from build123d import *

# Parameters (mm, degrees)
EXTRUDE_DEPTH   = 4
PAD_DEPTH       = 8
POCKET_START    = 4
SKETCH001_W     = 90
SKETCH001_H     = 4
POCKET_DEPTH    = 4
POCKET001_START = -5
SKETCH002_W     = 3.5
SKETCH002_H     = 1
SKETCH002_W_2   = 2.5
SKETCH002_H_2   = 3
SKETCH002_H_3   = 1.25
POCKET001_DEPTH = 89


with BuildPart() as part:
    # Face001 → Extrude (new body)
    with BuildSketch(Plane(origin=(44.07068, 49.485801, 0), x_dir=(0, 1, 0), z_dir=(0, 0, 1))):
        with BuildLine():
            add(Edge.make_bspline(
                [(-12.189347, 20.903638), (-8.616149, 10.816398)],
                knots=[0, 0, 8.089254, 8.089254], degree=1))
            add(Edge.make_bspline(
                [(-8.616149, 10.816398), (-9.34243, 10.514773)],
                knots=[0, 0, 0.594462, 0.594462], degree=1))
            add(Edge.make_bspline(
                [(-9.34243, 10.514773), (-9.595107, 10.410263), (-9.751211, 10.165523), (-9.751211, 9.903586)],
                knots=[0, 0, 0, 0, 1, 1, 1, 1], degree=3))
            add(Edge.make_bspline(
                [(-9.751211, 9.903586), (-9.751211, 9.842732), (-9.743274, 9.781877), (-9.724753, 9.7197)],
                knots=[0, 0, 0, 0, 1, 1, 1, 1], degree=3))
            add(Edge.make_bspline(
                [(-9.724753, 9.7197), (-6.950597, 0.094159)],
                knots=[0, 0, 7.572159, 7.572159], degree=1))
            add(Edge.make_bspline(
                [(-6.950597, 0.094159), (-7.703336, -0.194237)],
                knots=[0, 0, 0.609332, 0.609332], degree=1))
            add(Edge.make_bspline(
                [(-7.703336, -0.194237), (-7.963951, -0.292133), (-8.127992, -0.542164), (-8.127992, -0.809393)],
                knots=[0, 0, 0, 0, 1, 1, 1, 1], degree=3))
            add(Edge.make_bspline(
                [(-8.127992, -0.809393), (-8.127992, -0.874216), (-8.118732, -0.939039), (-8.098888, -1.003862)],
                knots=[0, 0, 0, 0, 1, 1, 1, 1], degree=3))
            add(Edge.make_bspline(
                [(-8.098888, -1.003862), (-2.807222, -18.201779)],
                knots=[0, 0, 13.601471, 13.601471], degree=1))
            add(Edge.make_bspline(
                [(-2.807222, -18.201779), (-2.752982, -18.37905), (-2.627305, -18.524571), (-2.460617, -18.603946)],
                knots=[0, 0, 0, 0, 1, 1, 1, 1], degree=3))
            add(Edge.make_bspline(
                [(-2.460617, -18.603946), (-2.29393, -18.683321), (-2.100784, -18.689935), (-1.930128, -18.621143)],
                knots=[0, 0, 0, 0, 1, 1, 1, 1], degree=3))
            add(Edge.make_bspline(
                [(-1.930128, -18.621143), (14.607653, -12.00656)],
                knots=[0, 0, 13.46384, 13.46384], degree=1))
            add(Edge.make_bspline(
                [(14.607653, -12.00656), (14.782278, -11.936446), (14.918539, -11.796216), (14.983362, -11.620268)],
                knots=[0, 0, 0, 0, 1, 1, 1, 1], degree=3))
            add(Edge.make_bspline(
                [(14.983362, -11.620268), (15.046862, -11.444321), (15.034956, -11.248529), (14.947643, -11.083164)],
                knots=[0, 0, 0, 0, 1, 1, 1, 1], degree=3))
            add(Edge.make_bspline(
                [(14.947643, -11.083164), (6.637081, 4.667482)],
                knots=[0, 0, 13.461663, 13.461663], degree=1))
            add(Edge.make_bspline(
                [(6.637081, 4.667482), (6.480976, 4.963815), (6.127758, 5.096107), (5.815549, 4.975721)],
                knots=[0, 0, 0, 0, 1, 1, 1, 1], degree=3))
            add(Edge.make_bspline(
                [(5.815549, 4.975721), (4.96756, 4.651607)],
                knots=[0, 0, 0.686226, 0.686226], degree=1))
            add(Edge.make_bspline(
                [(4.96756, 4.651607), (-0.018513, 13.744013)],
                knots=[0, 0, 7.83859, 7.83859], degree=1))
            add(Edge.make_bspline(
                [(-0.018513, 13.744013), (-0.181232, 14.041669), (-0.541065, 14.167346), (-0.851951, 14.0377)],
                knots=[0, 0, 0, 0, 1, 1, 1, 1], degree=3))
            add(Edge.make_bspline(
                [(-0.851951, 14.0377), (-1.578232, 13.736075)],
                knots=[0, 0, 0.594462, 0.594462], degree=1))
            add(Edge.make_bspline(
                [(-1.578232, 13.736075), (-6.192565, 23.392044)],
                knots=[0, 0, 8.089595, 8.089595], degree=1))
            add(Edge.make_bspline(
                [(-6.192565, 23.392044), (-6.344701, 23.709544), (-6.717763, 23.852419), (-7.043201, 23.717482)],
                knots=[0, 0, 0, 0, 1, 1, 1, 1], degree=3))
            add(Edge.make_bspline(
                [(-7.043201, 23.717482), (-11.81893, 21.735752)],
                knots=[0, 0, 3.908466, 3.908466], degree=1))
            add(Edge.make_bspline(
                [(-11.81893, 21.735752), (-12.07293, 21.629919), (-12.227711, 21.385179), (-12.227711, 21.124565)],
                knots=[0, 0, 0, 0, 1, 1, 1, 1], degree=3))
            add(Edge.make_bspline(
                [(-12.227711, 21.124565), (-12.227711, 21.050482), (-12.215805, 20.976398), (-12.189347, 20.903638)],
                knots=[0, 0, 0, 0, 1, 1, 1, 1], degree=3))
        make_face()
        with BuildLine():
            add(Edge.make_bspline(
                [(-24.664451, 2.497898), (-24.664451, 2.132773), (-24.368117, 1.83644), (-24.002992, 1.83644)],
                knots=[0, 0, 0, 0, 1, 1, 1, 1], degree=3))
            add(Edge.make_bspline(
                [(-24.002992, 1.83644), (-15.404034, 1.83644)],
                knots=[0, 0, 6.5, 6.5], degree=1))
            add(Edge.make_bspline(
                [(-15.404034, 1.83644), (-15.404034, -1.166581)],
                knots=[0, 0, 2.27, 2.27], degree=1))
            add(Edge.make_bspline(
                [(-15.404034, -1.166581), (-24.43294, -8.905643)],
                knots=[0, 0, 8.989056, 8.989056], degree=1))
            add(Edge.make_bspline(
                [(-24.43294, -8.905643), (-24.586399, -9.036612), (-24.664451, -9.221821), (-24.664451, -9.408352)],
                knots=[0, 0, 0, 0, 1, 1, 1, 1], degree=3))
            add(Edge.make_bspline(
                [(-24.664451, -9.408352), (-24.664451, -9.560487), (-24.611534, -9.713946), (-24.504378, -9.8383)],
                knots=[0, 0, 0, 0, 1, 1, 1, 1], degree=3))
            add(Edge.make_bspline(
                [(-24.504378, -9.8383), (-24.266253, -10.116112), (-23.849534, -10.147862), (-23.571722, -9.909737)],
                knots=[0, 0, 0, 0, 1, 1, 1, 1], degree=3))
            add(Edge.make_bspline(
                [(-23.571722, -9.909737), (-14.497836, -2.13231)],
                knots=[0, 0, 9.033744, 9.033744], degree=1))
            add(Edge.make_bspline(
                [(-14.497836, -2.13231), (-12.857419, -2.13231)],
                knots=[0, 0, 1.24, 1.24], degree=1))
            add(Edge.make_bspline(
                [(-12.857419, -2.13231), (-11.318867, -2.13231), (-10.112367, -0.970789), (-10.112367, 0.513523)],
                knots=[0, 0, 0, 0, 1, 1, 1, 1], degree=3))
            add(Edge.make_bspline(
                [(-10.112367, 0.513523), (-10.112367, 4.482273)],
                knots=[0, 0, 3, 3], degree=1))
            add(Edge.make_bspline(
                [(-10.112367, 4.482273), (-10.112367, 5.990398), (-11.250076, 7.128107), (-12.758201, 7.128107)],
                knots=[0, 0, 0, 0, 1, 1, 1, 1], degree=3))
            add(Edge.make_bspline(
                [(-12.758201, 7.128107), (-14.497836, 7.128107)],
                knots=[0, 0, 1.315, 1.315], degree=1))
            add(Edge.make_bspline(
                [(-14.497836, 7.128107), (-23.571722, 14.905534)],
                knots=[0, 0, 9.033744, 9.033744], degree=1))
            add(Edge.make_bspline(
                [(-23.571722, 14.905534), (-23.848211, 15.143659), (-24.266253, 15.111909), (-24.504378, 14.834096)],
                knots=[0, 0, 0, 0, 1, 1, 1, 1], degree=3))
            add(Edge.make_bspline(
                [(-24.504378, 14.834096), (-24.611534, 14.709742), (-24.664451, 14.556284), (-24.664451, 14.404148)],
                knots=[0, 0, 0, 0, 1, 1, 1, 1], degree=3))
            add(Edge.make_bspline(
                [(-24.664451, 14.404148), (-24.664451, 14.217617), (-24.586399, 14.032409), (-24.43294, 13.902763)],
                knots=[0, 0, 0, 0, 1, 1, 1, 1], degree=3))
            add(Edge.make_bspline(
                [(-24.43294, 13.902763), (-15.404034, 6.162377)],
                knots=[0, 0, 8.989707, 8.989707], degree=1))
            add(Edge.make_bspline(
                [(-15.404034, 6.162377), (-15.404034, 3.159357)],
                knots=[0, 0, 2.27, 2.27], degree=1))
            add(Edge.make_bspline(
                [(-15.404034, 3.159357), (-24.002992, 3.159357)],
                knots=[0, 0, 6.5, 6.5], degree=1))
            add(Edge.make_bspline(
                [(-24.002992, 3.159357), (-24.368117, 3.159357), (-24.664451, 2.863023), (-24.664451, 2.497898)],
                knots=[0, 0, 0, 0, 1, 1, 1, 1], degree=3))
        make_face()
        with BuildLine():
            add(Edge.make_bspline(
                [(17.253487, -13.990935), (17.593476, -13.854675), (17.757518, -13.468383), (17.622581, -13.131039)],
                knots=[0, 0, 0, 0, 1, 1, 1, 1], degree=3))
            add(Edge.make_bspline(
                [(17.622581, -13.131039), (17.48632, -12.792373), (17.101351, -12.627008), (16.762685, -12.761946)],
                knots=[0, 0, 0, 0, 1, 1, 1, 1], degree=3))
            add(Edge.make_bspline(
                [(16.762685, -12.761946), (-3.081065, -20.699446)],
                knots=[0, 0, 16.155494, 16.155494], degree=1))
            add(Edge.make_bspline(
                [(-3.081065, -20.699446), (-3.340357, -20.803956), (-3.497784, -21.052664), (-3.497784, -21.314602)],
                knots=[0, 0, 0, 0, 1, 1, 1, 1], degree=3))
            add(Edge.make_bspline(
                [(-3.497784, -21.314602), (-3.497784, -21.396623), (-3.483232, -21.479966), (-3.450159, -21.560664)],
                knots=[0, 0, 0, 0, 1, 1, 1, 1], degree=3))
            add(Edge.make_bspline(
                [(-3.450159, -21.560664), (-3.313899, -21.899331), (-2.92893, -22.064696), (-2.590263, -21.929758)],
                knots=[0, 0, 0, 0, 1, 1, 1, 1], degree=3))
            add(Edge.make_bspline(
                [(-2.590263, -21.929758), (17.253487, -13.990935)],
                knots=[0, 0, 16.155866, 16.155866], degree=1))
        make_face()
    extrude(amount=EXTRUDE_DEPTH)


with BuildPart() as part_1:
    # Extrude placement: moved
    add(part.part.moved(Location((2.348148, 3.053205, -2))))


with BuildPart() as part_2:
    # BaseFeature placement: moved
    add(part_1.part.moved(Location((-2.348148, -3.053205, 2))))

    # Sketch → Pad (new body)
    with BuildSketch(Plane.XY):
        with BuildLine():
            Line((0, 98), (0, 5))
            ThreePointArc((0, 5), (1.464466, 1.464466), (5, 0))
            Line((5, 0), (85, 0))
            ThreePointArc((85, 0), (88.535534, 1.464466), (90, 5))
            Line((90, 5), (90, 98))
            Line((90, 98), (0, 98))
        make_face()
    extrude(amount=PAD_DEPTH)

    # Sketch001 → Pocket (cut)
    with BuildSketch(Plane.XY.offset(POCKET_START)):
        with BuildLine():
            Line((4.5, 98), (4.5, 5))
            ThreePointArc((4.5, 5), (4.792893, 4.292893), (5.5, 4))
            Line((5.5, 4), (84.5, 4))
            ThreePointArc((84.5, 4), (85.207107, 4.292893), (85.5, 5))
            Line((85.5, 5), (85.5, 98))
            Line((85.5, 98), (4.5, 98))
        make_face()
        with Locations((45, 96)):
            Rectangle(SKETCH001_W, SKETCH001_H)
    extrude(amount=POCKET_DEPTH, mode=Mode.SUBTRACT)

    # Sketch002 → Pocket001 (cut)
    with BuildSketch(Plane.XZ.offset(POCKET001_START)):
        with Locations((87.75, 4.5)):
            Rectangle(SKETCH002_W, SKETCH002_H)
        with Locations((87.75, 6.5)):
            Rectangle(SKETCH002_W_2, SKETCH002_H_2)
        with Locations((2.25, 4.375)):
            Rectangle(SKETCH002_W, SKETCH002_H_3)
        with Locations((2.25, 6.5)):
            Rectangle(SKETCH002_W_2, SKETCH002_H_2)
    extrude(amount=-POCKET001_DEPTH, mode=Mode.SUBTRACT)


solid = part_2.part
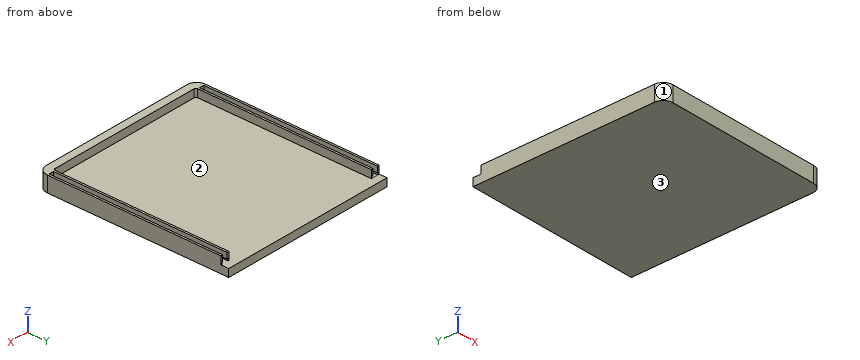
CAD build for the part. Positions are in the model's coordinates, mm. Face numbers are marked on the shaded views. Coordinates: 2 decimals unless noted, no trailing zeros. Write each loop counter-clockwise with the first axis right and the second up, starting at its lowest first coordinate (ties: lowest second). Pieces come first, ordered by that corner, then holes. Notation, with made-up numbers: M 86,26 L 97,26 A21 cw 97,51 Z; hole C -32.5,15 d6. An arc over 180 degrees is marked long. Return JSON: item names as keys, results as strings.
Item 1: Slice it at A-A, the plane z = 6.25. Write the cut outline in (x, y), and give its area (3 significant figures).
Findings below:
{"outline": "M 0,5 A5 ccw 5,0 L 85,0 A5 ccw 90,5 L 90,94 L 89,94 L 89,5 L 86.5,5 L 86.5,94 L 85.5,94 L 85.5,5 A1 cw 84.5,4 L 5.5,4 A1 cw 4.5,5 L 4.5,94 L 3.5,94 L 3.5,5 L 1,5 L 1,94 L 0,94 Z", "area": "715 mm2"}
Item 2: Drop flat-ended pins along their axis: pin 1 Ø4 at (x, z) = (87.5, 6.5) entering from +Y; pin 2 Ø2 at (x, z) = (27, 7) entering from +Y; pin 3 Ø2 at (x, y) = (10, 60.5) entering from +Z. Give the stop position or say it passes through.
Findings below:
{"pin 1": "stops at y = 94", "pin 2": "stops at y = 4", "pin 3": "stops at z = 4"}
Item 3: Two-plate mould, pull along X, no slides. Class the marked faces 1, 2 and 3: +X half, -X half, draft (parallel to the pull), parting line (faces both ways), or undercut.
Findings below:
{"face 1": "-X half", "face 2": "undercut", "face 3": "draft"}
Item 4: Slice it at B-B, the plane y = 79. Write the cut outline in (x, z), and give its area (3 significant figures).
Findings below:
{"outline": "M 0,0 L 90,0 L 90,8 L 89,8 L 89,5 L 89.5,5 L 89.5,4 L 86,4 L 86,5 L 86.5,5 L 86.5,8 L 85.5,8 L 85.5,4 L 4.5,4 L 4.5,8 L 3.5,8 L 3.5,5 L 4,5 L 4,3.75 L 0.5,3.75 L 0.5,5 L 1,5 L 1,8 L 0,8 Z", "area": "373 mm2"}
Item 5: Slice it at C-C, the plane x = 19. Write the cut outline in (y, z).
Findings below:
{"outline": "M 0,0 L 98,0 L 98,4 L 4,4 L 4,8 L 0,8 Z"}
Item 6: Probe line 1 (X direction, y = 91.5, z = 6); line 2 (Z direction, x = 46, y = 12). List the from-to ranges inside material, lowest first. Write a range as from..to.
Findings below:
{"line 1": "x = 0..1, 3.5..4.5, 85.5..86.5, 89..90", "line 2": "z = 0..4"}
